Here's the drawing with two shaded views (mm, measured from the low corner). I have some questions. A direction names the side the tool comes from. Round coordinates to 2 decimals unless told otherwise and drop trailing zeros. Loops run counter-clockwise (first coordinate to the right, second up) from the corner with the lowest first, then second, coordinate; pieces in that order, holes last.
(1) Will these pins go through, and if not, where does the flat tip stop? pin 1 Ø1 at (x, z) = (57, 25) entering from -Y; pin 2 Ø1 at (x, y) = (82.5, 26) entering from +Z; pin 3 Ø10 at (y, z) = (18.5, 17.5) entering from -X; pin 4 Ø5 at (x, z) = (104, 26.5) entering from -Y.
(2) I want a section at A-A on z = 67. Write out the boundary of the cut face in (x, y), plus the area to 3 significant figures.
(3) I want a section at D-D on x = 33. Write out the boundary of the cut face in (y, z), plus the area to 3 significant figures.
(4) I want a section at C-C on z = 44. Write out the boundary of the cut face in (x, y), plus the area to 4 significant figures.
(5) If I drill on line 1 along X through (y, z) = (44.5, 63); line 2 along X through (y, z) = (12, 39.5); line 3 along Z through (x, y) = (96, 40.5), over which ranges is the centre line in solid material (lowest first)?
(6) Thinking about a two-plate mould opening in X: for the marked faces 1, 2 and 3, which applies, released by +X, released by -X, zero draft, split by the parting line, or undercut?
(7) Which directions (+Z, -Z, +X, -X, +Y, -Y) give clear straight access to the entire face, cutting with the end or side of a thin tool? Please do the marked faces 4, 5, 6, 7 and 8.
(8) I want a section at B-B on y = 21. Write out the boundary of the cut face in (x, z), plus the area to 3 significant figures.
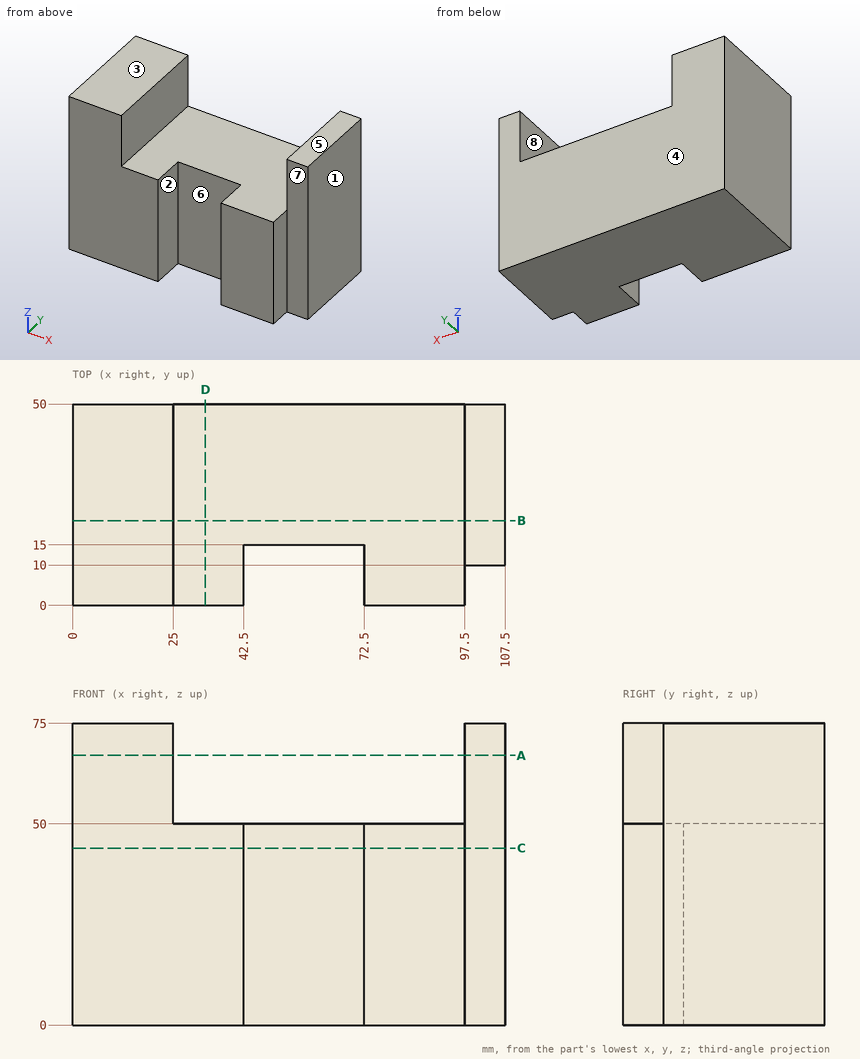
Filled sheet:
1. pin 1: stops at y = 15
1. pin 2: stops at z = 50
1. pin 3: stops at x = 0
1. pin 4: stops at y = 10
2. outline: (0, 0) - (25, 0) - (25, 50) - (0, 50) - close; (97.5, 10) - (107.5, 10) - (107.5, 50) - (97.5, 50) - close
2. area: 1,650 mm2
3. outline: (0, 0) - (50, 0) - (50, 50) - (0, 50) - close
3. area: 2,500 mm2
4. outline: (0, 0) - (42.5, 0) - (42.5, 15) - (72.5, 15) - (72.5, 0) - (97.5, 0) - (97.5, 10) - (107.5, 10) - (107.5, 50) - (0, 50) - close
4. area: 4,825 mm2
5. line 1: x = 0 to 25, 97.5 to 107.5
5. line 2: x = 0 to 42.5, 72.5 to 107.5
5. line 3: z = 0 to 50
6. face 1: released by +X
6. face 2: undercut
6. face 3: zero draft
7. face 4: +Z, -Z, +X, -X, +Y
7. face 5: +Z, +X, -X, +Y, -Y
7. face 6: +Z, -Z, -Y
7. face 7: +Z, -Z, +X, -Y
7. face 8: +Z, +Y, -Y
8. outline: (0, 0) - (107.5, 0) - (107.5, 75) - (97.5, 75) - (97.5, 50) - (25, 50) - (25, 75) - (0, 75) - close
8. area: 6,250 mm2
